Verification items for the finished model (mm, model axes). Face numbers are marked on the shaded views. Coordinates: 2 decimals unless noted, no trailing zeros. Loops run counter-clockwise (first coordinate to the right, second up) from the corner with the lowest first, then second, coordinate; pieces in that order, holes last.
Q1. Mould release check, pull along X, two halves, no side actions. Record for the marked faces 1, 2 and 3: +X half, -X half, draft (parallel to the pull), parting line (faces both ways), or undercut.
Q2. Sectioned sample at A-A (x = 0). Enter the section's corners in (y, z).
Q3. Sectioned sample at C-C (y = 5.5). Enter the section's corners in (x, z).
Q4. Go/stop test with flat-tipped pins: P1, Ø1.5, axis at x = 0, y = 34, coming from the +Z side; P2, Ø13, axis at x = 10, z = 6, coming from the +Y side; P3, Ø5, axis at y = 61.5, z = -4.5, coming from the +X side. Record where each tip stops, or that it passes through.
Q5. Material ranges on probe 1 along Z at (x, y) = (0, 42); probe 2 along Y at (x, z) = (9, -16); probe 3 along Z at (x, y) = (10, 53.5), recorded low to high.
Q6. Sectioned sample at B-B (z = 0). Enter the section's corners in (x, y).
```python
from build123d import *

# Parameters (mm, degrees)
SKETCH1_R           = 22.5
SKETCH1_R_2         = 21.5
EXTRUDE_THIN1_DEPTH = 70
SKETCH1_3_R         = 21.5
BOSS_EXTRUDE1_DEPTH = 1
FILLET1_R           = 3
SKETCH2_R           = 1.5
CUT_EXTRUDE1_DEPTH  = 1


with BuildPart() as part:
    # Sketch1 → Extrude-Thin1 (new body)
    with BuildSketch(Plane(origin=(0, 0, 0), x_dir=(1, 0, 0), z_dir=(0, 1, 0))):
        Circle(SKETCH1_R)
        Circle(SKETCH1_R_2, mode=Mode.SUBTRACT)
    extrude(amount=EXTRUDE_THIN1_DEPTH)

    # Sketch1<3> → Boss-Extrude1 (add)
    with BuildSketch(Plane(origin=(0, 0, 0), x_dir=(1, 0, 0), z_dir=(0, 1, 0))):
        Circle(SKETCH1_3_R)
    extrude(amount=BOSS_EXTRUDE1_DEPTH)

    # Fillet1
    fillet1_edges = [part.edges().sort_by_distance(p)[0] for p in [
        (-22.5, 0, 0),
    ]]
    fillet(fillet1_edges, radius=FILLET1_R)

    # Sketch2 → Cut-Extrude1 (cut)
    with BuildSketch(Plane.XZ):
        with Locations(Location((0, 0, 0), (0, 0, 270))):
            Circle(SKETCH2_R)
    extrude(amount=-CUT_EXTRUDE1_DEPTH, mode=Mode.SUBTRACT)


solid = part.part
```
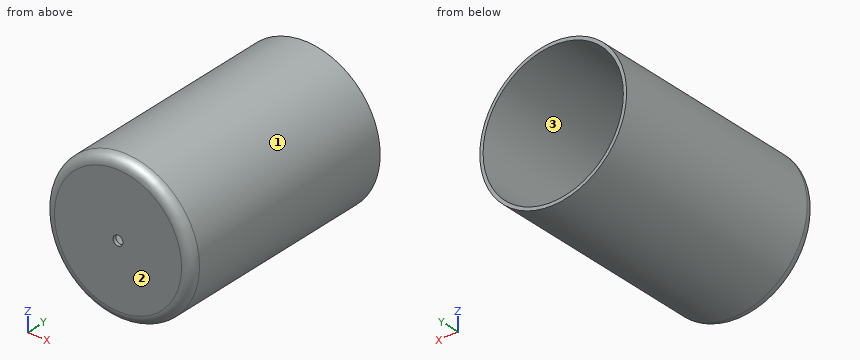
Geometry check:
1. face 1: parting line
1. face 2: draft
1. face 3: undercut
2. outline: (0, -19.5) arc R3 ccw to (3, -22.5) - (70, -22.5) - (70, -21.5) - (1, -21.5) - (1, -1.5) - (0, -1.5) - close; (0, 1.5) - (1, 1.5) - (1, 21.5) - (70, 21.5) - (70, 22.5) - (3, 22.5) arc R3 ccw to (0, 19.5) - close
3. outline: circle Ø45 at (0, 0); hole circle Ø43 at (0, 0)
4. P1: stops at z = 22.5
4. P2: stops at y = 1
4. P3: stops at x = 22.41
5. probe 1: z = -22.5 to -21.5, 21.5 to 22.5
5. probe 2: y = 0 to 1
5. probe 3: z = -20.16 to -19.03, 19.03 to 20.16
6. outline: (-22.5, 3) arc R3 ccw to (-19.5, 0) - (-1.5, 0) - (-1.5, 1) - (-21.5, 1) - (-21.5, 70) - (-22.5, 70) - close; (1.5, 0) - (19.5, 0) arc R3 ccw to (22.5, 3) - (22.5, 70) - (21.5, 70) - (21.5, 1) - (1.5, 1) - close
